Geometry check sheet. Reference: drawing and pictorial views, mm from the part's lowest x, y, z. A direction names the side the tool comes from. Round coordinates to 2 decimals unless told otherwise and drop trailing zeros. Loops run counter-clockwise (first coordinate to the right, second up) from the corner with the lowest first, then second, coordinate; pieces in that order, holes last. Notation, with made-up numbers: (-9, 59.5) - (11, 59.5) arc R26 cw to (11, 87.5) - close; hole circle Ø9 at (5, 80). An arc over 180 degrees is marked (long way). Answer in a Markdown table with one row per item. Add a question column.
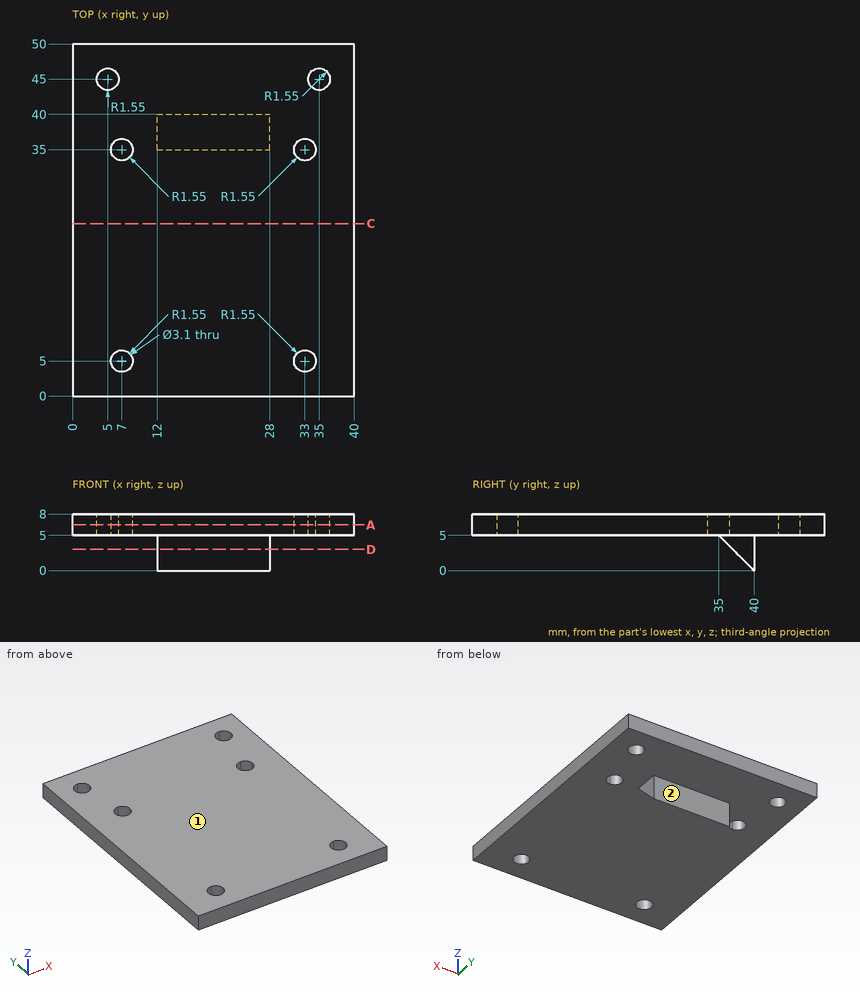
Q1. Set-up check for the marked faces 1 and 2: record each of +Z, -Z, +X, -X, +Y, -Y from which the full face is reachable in a straight line by a thin tool's end or side.
Q2. Scan lines: line 1 (Y direction, x = 7, z = 6.4); line 2 (X direction, y = 5, z = 6.5); line 3 (Z direction, x = 8, y = 41). Record each from-to range of solid material in increasing order. Write a range as from..to.
Q3. Cross-section at D-D, the plane z = 3. Enter the section's corners in (x, y).
Q4. Cross-section at A-A, the plane z = 6.5. Enter the section's corners in (x, y), plus the area to 3 significant figures.
Q5. Cross-section at C-C, the plane y = 24.5. Enter the section's corners in (x, z), plus the area to 3 significant figures.
Q6. Depth check by flat-ended pin: P1, Ø2, axis at x = 31, y = 41, coming from the -Z side; P2, Ø1.5, axis at x = 16.5, z = 3.5, coming from the +Y side; P3, Ø4, axis at y = 37, z = 2.5, coming from the +X side. Enter the tip coordinate at first touch or a pass-through.
Check sheet entries:
| question | item | result |
|---|---|---|
| 1 | face 1 | +Z, +X, -X, +Y, -Y |
| 1 | face 2 | -Z, +X, -X, +Y |
| 2 | line 1 | 0..3.45, 6.55..33.45, 36.55..50 |
| 2 | line 2 | 0..5.45, 8.55..31.45, 34.55..40 |
| 2 | line 3 | 5..8 |
| 3 | outline | (12, 37) - (28, 37) - (28, 40) - (12, 40) - close |
| 4 | outline | (0, 0) - (40, 0) - (40, 50) - (0, 50) - close; hole circle Ø3.1 at (5, 45); hole circle Ø3.1 at (7, 5); hole circle Ø3.1 at (7, 35); hole circle Ø3.1 at (33, 5); hole circle Ø3.1 at (33, 35); hole circle Ø3.1 at (35, 45) |
| 4 | area | 1,950 mm² |
| 5 | outline | (0, 5) - (40, 5) - (40, 8) - (0, 8) - close |
| 5 | area | 120 mm² |
| 6 | P1 | z = 5 |
| 6 | P2 | y = 40 |
| 6 | P3 | x = 28 |
